Verification items for the finished model (mm, model axes). A direction names the side the tool comes from. Coordinates: 2 decimals unless noted, no trailing zeros. Write each loop counter-clockwise with the first axis right and the second up, starting at its lowest first coordinate (ties: lowest second). Pieces come first, ordered by that corner, then holes. Notation, with made-up numbers: (-10, 68.5) -> (7, 68.5) arc R32 ccw to (7, 102.5) -> close; hole circle Ø1 at (47, 5). An arc over 180 degrees is marked (long way). Answer in a Markdown table with one row per item.
```python
from build123d import *

# Parameters (mm, degrees)
BOSS_EXTRUDE1_DEPTH      = 2
CUT_EXTRUDE1_REACH       = 27.75
SKETCH2_R                = 1.7145
SKETCH3_R                = 1.7145
BOSS_EXTRUDE2_DEPTH      = 72.305
CUT_EXTRUDE2_REACH       = 78.727
SKETCH4_R                = 8.99
BOSS_EXTRUDE3_DEPTH      = 2
BOSS_EXTRUDE3_DEPTH_BACK = 2
SKETCH5_R                = 21
SKETCH5_R_2              = 8.99
CUT_EXTRUDE3_DEPTH       = 2
SKETCH7_R                = 21
SKETCH7_R_2              = 8.99
BOSS_EXTRUDE4_DEPTH      = 2
SKETCH8_R                = 1.7145
BOSS_EXTRUDE5_DEPTH      = 57.305


with BuildPart() as part:
    # Sketch1 → Boss-Extrude1 (new body)
    with BuildSketch(Plane(origin=(0, 0, 0), x_dir=(1, 0, 0), z_dir=(0, 1, 0))):
        with BuildLine():
            Line((-2.743211684, 13.490721697), (-2.743211684, 19.02714))
            Line((-2.743211684, 19.02714), (0.674160958, 19.02714))
            Line((0.674160958, 19.02714), (0.674160958, 13.750283242))
            ThreePointArc((0.674160958, 13.750283242), (8.929745908, 10.47780608), (13.469544487, 2.845374062))
            ThreePointArc((13.469544487, 2.845374062), (17.232722938, 0.513379028), (13.615039655, -2.03849882))
            ThreePointArc((13.615039655, -2.03849882), (9.237791247, -10.207252084), (0.674160958, -13.750283242))
            Line((0.674160958, -13.750283242), (0.674160958, -15.99946))
            Line((0.674160958, -15.99946), (-2.743211684, -15.99946))
            Line((-2.743211684, -15.99946), (-2.743211684, -13.490721697))
            ThreePointArc((-2.743211684, -13.490721697), (-9.966316815, -9.49722651), (-13.607209812, -2.090125207))
            ThreePointArc((-13.607209812, -2.090125207), (-17.080297956, 0.514213195), (-13.456831252, 2.904905316))
            ThreePointArc((-13.456831252, 2.904905316), (-9.676012861, 9.792831937), (-2.743211684, 13.490721697))
        make_face()
    extrude(amount=-BOSS_EXTRUDE1_DEPTH)

    # Sketch2 → Cut-Extrude1 (cut, up to next)
    with BuildSketch(Plane(origin=(0, 0, 0), x_dir=(1, 0, 0), z_dir=(0, 1, 0)), mode=Mode.PRIVATE) as cut_extrude1_sk1:
        with Locations(Location((14.5796, 0.43434, 0), (0, 0, 270))):
            Circle(SKETCH2_R)
    cut_extrude1_tool1 = extrude(cut_extrude1_sk1.sketch, amount=-CUT_EXTRUDE1_REACH, mode=Mode.PRIVATE) & part.part
    # Sketch2 → Cut-Extrude1 (cut, up to next)
    with BuildSketch(Plane(origin=(0, 0, 0), x_dir=(1, 0, 0), z_dir=(0, 1, 0)), mode=Mode.PRIVATE) as cut_extrude1_sk2:
        with Locations(Location((-14.4272, 0.43434, 0), (0, 0, 270))):
            Circle(SKETCH2_R)
    cut_extrude1_tool2 = extrude(cut_extrude1_sk2.sketch, amount=-CUT_EXTRUDE1_REACH, mode=Mode.PRIVATE) & part.part
    add(cut_extrude1_tool1.solids().sort_by_distance((14.5796, 0, -0.43434))[0], mode=Mode.SUBTRACT)
    add(cut_extrude1_tool2.solids().sort_by_distance((-14.4272, 0, -0.43434))[0], mode=Mode.SUBTRACT)

    # Sketch3 → Boss-Extrude2 (add)
    # profile 1 of 2: a face of its own
    with BuildSketch(Plane.XZ.offset(2)):
        with BuildLine():
            ThreePointArc((13.469544487, -2.845374062), (16.011187954, -2.669483042), (17.2339, -0.43434))
            ThreePointArc((17.2339, -0.43434), (16.077110595, 1.757182418), (13.615039655, 2.03849882))
            ThreePointArc((13.615039655, 2.03849882), (11.926477062, -0.355300972), (13.469544487, -2.845374062))
        make_face()
        with Locations(Location((14.5796, -0.43434, 0), (0, 0, 90))):
            Circle(SKETCH3_R, mode=Mode.SUBTRACT)
    # profile 2 of 2: a face of its own
    with BuildSketch(Plane.XZ.offset(2)):
        with BuildLine():
            ThreePointArc((-13.456831252, -2.904905316), (-12.233919551, -1.929274567), (-11.7729, -0.43434))
            ThreePointArc((-11.7729, -0.43434), (-12.279898386, 1.125917756), (-13.607209812, 2.090125207))
            ThreePointArc((-13.607209812, 2.090125207), (-17.080297956, -0.514213195), (-13.456831252, -2.904905316))
        make_face()
        with Locations(Location((-14.4272, -0.43434, 0), (0, 0, 90))):
            Circle(SKETCH3_R, mode=Mode.SUBTRACT)
    extrude(amount=BOSS_EXTRUDE2_DEPTH)

    # Sketch4 → Cut-Extrude2 (cut, up to next)
    with BuildSketch(Plane.XZ.offset(2), mode=Mode.PRIVATE) as cut_extrude2_sk1:
        with Locations(Location((0, 0, 0), (0, 0, 270))):
            Circle(SKETCH4_R)
    cut_extrude2_tool1 = extrude(cut_extrude2_sk1.sketch, amount=-CUT_EXTRUDE2_REACH, mode=Mode.PRIVATE) & part.part
    add(cut_extrude2_tool1.solids().sort_by_distance((0, -2, 0))[0], mode=Mode.SUBTRACT)

    # Sketch5 → Boss-Extrude3 (add, two sides: drawn at the far end of the back side and taken through both)
    with BuildSketch(Plane.XZ.offset(74.305).offset(-BOSS_EXTRUDE3_DEPTH_BACK)):
        with Locations(Location((0, 0, 0), (0, 0, 270))):
            Circle(SKETCH5_R)
        with Locations(Location((0, 0, 0), (0, 0, 270))):
            Circle(SKETCH5_R_2, mode=Mode.SUBTRACT)
    extrude(amount=BOSS_EXTRUDE3_DEPTH + BOSS_EXTRUDE3_DEPTH_BACK)

    # Sketch6 → Cut-Extrude3 (cut)
    with BuildSketch(Plane.XZ.offset(76.305)):
        with BuildLine():
            Line((-7.35, 13.65), (-10, 0))
            Line((-10, 0), (-7.35, -13.65))
            ThreePointArc((-7.35, -13.65), (0, -15.503480297), (7.35, -13.65))
            Line((7.35, -13.65), (10, 0))
            Line((10, 0), (7.35, 13.65))
            ThreePointArc((7.35, 13.65), (0, 15.503480297), (-7.35, 13.65))
        make_face()
    extrude(amount=-CUT_EXTRUDE3_DEPTH, mode=Mode.SUBTRACT)

    # Sketch7 → Boss-Extrude4 (add)
    with BuildSketch(Plane(origin=(0, -37.305, 0), x_dir=(1, 0, 0), z_dir=(0, 1, 0))):
        with Locations(Location((0, 0, 0), (0, 0, 90))):
            Circle(SKETCH7_R)
        with Locations(Location((0, 0, 0), (0, 0, 90))):
            Circle(SKETCH7_R_2, mode=Mode.SUBTRACT)
    extrude(amount=BOSS_EXTRUDE4_DEPTH)

    # Sketch8 → Boss-Extrude5 (add)
    with BuildSketch(Plane(origin=(0, -72.305, 0), x_dir=(1, 0, 0), z_dir=(0, 1, 0))):
        with Locations(Location((-14.4272, 0.43434, 0), (0, 0, 270))):
            Circle(SKETCH8_R)
        with Locations(Location((14.5796, 0.43434, 0), (0, 0, 270))):
            Circle(SKETCH8_R)
    extrude(amount=BOSS_EXTRUDE5_DEPTH)


solid = part.part
```
1. Tool access check on faces 5 (the flat face through (-14, -15, 0)), 6 (the cylindrical face through (-0.107, -75.319, -15.503)), 7 (the flat face through (0.674, -1, 15)), 8 (the flat face through (0.674, -1, -16)). Record the directions out of +Z, -Z, +X, -X, +Y, -Y that give a thin tool (end or side, any length) a straight path to the whole face; none if there is none.
Geometry says:
| item | result |
|---|---|
| face 5 | +Y |
| face 6 | -Y |
| face 7 | +Z, +X, +Y |
| face 8 | -Z, +X, +Y |
2. Section check C-C, the plane z = 18.5. Record the boundary of the cut face in (x, y) (3 decimals), plus the area to 3 significant figures.
Geometry says:
| item | result |
|---|---|
| outline | (-9.937, -76.305) -> (9.937, -76.305) -> (9.937, -72.305) -> (-9.937, -72.305) -> close; (-9.937, -37.305) -> (9.937, -37.305) -> (9.937, -35.305) -> (-9.937, -35.305) -> close |
| area | 119 mm^2 |
3. Section check D-D, the plane y = -20.5. Record the boundary of the cut face in (x, z).
Geometry says:
| item | result |
|---|---|
| outline | circle Ø5.31 at (-14.43, -0.43); circle Ø5.31 at (14.58, -0.43) |
4. Thickness scan on line 1 (Y direction, x = 5.5, z = 12) (3 decimals); line 2 (Y direction, x = 4.5, z = -16) (3 decimals); line 3 (X direction, y = -36, z = 0). Record the ranges inside material, lowest first. Write a range as from..to.
Geometry says:
| item | result |
|---|---|
| line 1 | -74.305..-72.305, -37.305..-35.305, -2..0 |
| line 2 | -76.305..-72.305, -37.305..-35.305 |
| line 3 | -21..-8.99, 8.99..21 |
5. Depth check by flat-ended pin: P1, Ø1, axis at y = -1.5, z = 14.5, coming from the -X side; P2, Ø12, axis at y = -59, z = 1.5, coming from the +X side; P3, Ø10, axis at x = -1, z = -4, coming from the -Y side (3 decimals). Enter the tip coordinate at first touch or a pass-through.
Geometry says:
| item | result |
|---|---|
| P1 | x = -2.74 |
| P2 | x = 17.23 |
| P3 | y = -74.305 |
6. Section check A-A, the plane z = -4.5. Record the boundary of the cut face in (x, y) (3 decimals).
Geometry says:
| item | result |
|---|---|
| outline | (-20.512, -76.305) -> (-9.126, -76.305) -> (-9.126, -74.305) -> (-7.783, -74.305) -> (-7.783, -72.305) -> (-20.512, -72.305) -> close; (-20.512, -37.305) -> (-7.783, -37.305) -> (-7.783, -35.305) -> (-20.512, -35.305) -> close; (-13.011, -2) -> (-7.783, -2) -> (-7.783, 0) -> (-13.011, 0) -> close; (7.783, -74.305) -> (9.126, -74.305) -> (9.126, -76.305) -> (20.512, -76.305) -> (20.512, -72.305) -> (7.783, -72.305) -> close; (7.783, -37.305) -> (20.512, -37.305) -> (20.512, -35.305) -> (7.783, -35.305) -> close; (7.783, -2) -> (13.011, -2) -> (13.011, 0) -> (7.783, 0) -> close |
7. Section check B-B, the plane x = -6.5. Record the boundary of the cut face in (y, z) (3 decimals).
Geometry says:
| item | result |
|---|---|
| outline | (-76.305, -19.969) -> (-72.305, -19.969) -> (-72.305, -6.21) -> (-74.305, -6.21) -> (-74.305, -14.075) -> (-76.305, -14.075) -> close; (-76.305, 14.075) -> (-74.305, 14.075) -> (-74.305, 6.21) -> (-72.305, 6.21) -> (-72.305, 19.969) -> (-76.305, 19.969) -> close; (-37.305, -19.969) -> (-35.305, -19.969) -> (-35.305, -6.21) -> (-37.305, -6.21) -> close; (-37.305, 6.21) -> (-35.305, 6.21) -> (-35.305, 19.969) -> (-37.305, 19.969) -> close; (-2, -12.136) -> (0, -12.136) -> (0, -6.21) -> (-2, -6.21) -> close; (-2, 6.21) -> (0, 6.21) -> (0, 12.136) -> (-2, 12.136) -> close |
8. Mould release check, pull along Z, two halves, no side actions. Record for faces 1 (the flat face through (-1, -1, -19.027)), 2 (the cylindrical face through (-6.31, -36.32, -20.03)), 3 (the flat face through (-1, -1, 15.999)), 4 (the flat face through (8.7, -75.3, 6.7)): released by +Z, released by -Z, zero draft, split by the parting line, or undercut.
Geometry says:
| item | result |
|---|---|
| face 1 | released by -Z |
| face 2 | split by the parting line |
| face 3 | released by +Z |
| face 4 | undercut |
